Could you check a few things on this model? Use its own coordinates, in mm. A direction names the side the tool comes from. Round coordinates to 2 decimals unless told otherwise and drop trailing zeros. Order: outer loops, then holes, each group sorted by start corner. A loop starts at its lowest first (then second) coordinate and runs counter-clockwise, first axis right, second up. Notation, with made-up numbers: (-1.75, -5.75) -> (26.25, -5.75) arc R31 cw to (26.25, 32.25) -> close; hole circle Ø6 at (-18, 81.5). An arc over 180 degrees is marked (long way). One line per question, with ' | ' between items.
```python
from build123d import *

# Parameters (mm, degrees)
F0_W     = 10
F0_H     = 50
F1_DEPTH = 5.4
F3_START = 4.6
F2_W     = 8.5828267038
F2_H     = 11.0100731254
F2_W_2   = 12.8774824552
F2_H_2   = 6.9046204444
F2_W_3   = 25.3804451786
F2_H_3   = 7.8376773745
F2_H_4   = 6.3447866123
F2_W_4   = 17.729378771
F3_DEPTH = 4.8


with BuildPart() as f1:
    # F0 (on Front) → F1 (new body)
    with BuildSketch(Plane.XZ):
        Rectangle(F0_W, F0_H)
    extrude(amount=F1_DEPTH)

    # F2 (on Front) → F3 (join)
    with BuildSketch(Plane.XZ.offset(F3_START)):
        with Locations((-0.4671770148, 19.0343614668)):
            Rectangle(F2_W, F2_H)
        with Locations((10.2629775647, 19.0343614668)):
            Rectangle(F2_W_2, F2_H)
        with Locations((-0.4671770148, -7.2778436588)):
            Rectangle(F2_W, F2_H_2)
        with Locations((16.5144589264, -7.2778436588)):
            Rectangle(F2_W_3, F2_H_2)
        with Locations((-0.4671770148, -18.7544440851)):
            Rectangle(F2_W, F2_H_3)
        Polygon((3.8242363371, -14.7295454517), (3.8242363371, -14.8356053978), (3.8242363371, -22.6732827723), (43.2005375624, -22.6732827723), (43.2005375624, -14.7295454517), align=None)
        with Locations((-0.4671770148, 6.6247038776)):
            Rectangle(F2_W, F2_H_4)
        with Locations((12.6889257226, 6.6247038776)):
            Rectangle(F2_W_4, F2_H_4)
    extrude(amount=F3_DEPTH)


solid = f1.part
```
1. I want a section at C-C on y = -6.5. List the corners of the cut face in (x, z) for me.
From the geometry:
outline: (-4.76, -22.67) -> (43.2, -22.67) -> (43.2, -14.73) -> (3.82, -14.73) -> (3.82, -14.84) -> (-4.76, -14.84) -> close; (-4.76, -10.73) -> (29.2, -10.73) -> (29.2, -3.83) -> (-4.76, -3.83) -> close; (-4.76, 3.45) -> (21.55, 3.45) -> (21.55, 9.8) -> (-4.76, 9.8) -> close; (-4.76, 13.53) -> (16.7, 13.53) -> (16.7, 24.54) -> (-4.76, 24.54) -> close
2. I want a section at A-A on x = 18.5. List the corners of the cut face in (y, z) for me, and give its area (3 significant figures).
From the geometry:
outline: (-9.4, -22.67) -> (-4.6, -22.67) -> (-4.6, -14.73) -> (-9.4, -14.73) -> close; (-9.4, -10.73) -> (-4.6, -10.73) -> (-4.6, -3.83) -> (-9.4, -3.83) -> close; (-9.4, 3.45) -> (-4.6, 3.45) -> (-4.6, 9.8) -> (-9.4, 9.8) -> close | area: 102 mm²
3. I want a section at B-B on x = 13.5. List the corners of the cut face in (y, z) for me, and give its area (3 significant figures).
From the geometry:
outline: (-9.4, -22.67) -> (-4.6, -22.67) -> (-4.6, -14.73) -> (-9.4, -14.73) -> close; (-9.4, -10.73) -> (-4.6, -10.73) -> (-4.6, -3.83) -> (-9.4, -3.83) -> close; (-9.4, 3.45) -> (-4.6, 3.45) -> (-4.6, 9.8) -> (-9.4, 9.8) -> close; (-9.4, 13.53) -> (-4.6, 13.53) -> (-4.6, 24.54) -> (-9.4, 24.54) -> close | area: 155 mm²
4. I want a section at D-D on z = 21. List the corners of the cut face in (x, y) for me, and give its area (3 significant figures).
From the geometry:
outline: (-5, -5.4) -> (-4.76, -5.4) -> (-4.76, -9.4) -> (16.7, -9.4) -> (16.7, -4.6) -> (5, -4.6) -> (5, 0) -> (-5, 0) -> close | area: 149 mm²
5. If we mould it in two halves opening along Z, with no side actions, what happens to faces 1 (the face through (0, -3, 25)), 2 (the face through (16.702, -7, 19)), 3 (the face through (9, -7, 9.797)), 4 (the face through (-1, -7, -14.836))? For each: pulls with the +Z half, pulls with the -Z half, needs draft (parallel to the pull), parting line crosses it, or undercut.
From the geometry:
face 1: pulls with the +Z half | face 2: needs draft | face 3: undercut | face 4: undercut
6. I'm going to push flat-ended pins straight in: pin 1 (1.4 mm diameter, centred on x = 3, y = -6, fed in from -Z); pin 2 (2.5 mm diameter, centred on x = 23, y = -6.5, fed in from -Z); pin 3 (2 mm diameter, centred on y = -8, z = 6.5, fed in from -X); pin 4 (3.5 mm diameter, centred on x = 23, z = -8, fed in from +Y). Where does each tip first touch, or does it pass through?
From the geometry:
pin 1: stops at z = -25 | pin 2: stops at z = -22.67 | pin 3: stops at x = -4.76 | pin 4: stops at y = -4.6
7. I need wall thicknesses on probe 1 along Z at (x, y) = (19, -5.75); probe 2 along Z at (x, y) = (26.5, -7.5); probe 3 along Z at (x, y) = (16.5, -6). Which ranges of each line are inside material? Lowest first, please.
From the geometry:
probe 1: z = -22.67 to -14.73, -10.73 to -3.83, 3.45 to 9.8 | probe 2: z = -22.67 to -14.73, -10.73 to -3.83 | probe 3: z = -22.67 to -14.73, -10.73 to -3.83, 3.45 to 9.8, 13.53 to 24.54
8. On a 3-axis mill with a long thin cutter (end or side, diameter ignored), from which of +Z, -Z, +X, -X, +Y, -Y can I reach the whole of each face in a straight line? I mean faces 5 (the face through (24, -4.6, -19)), 6 (the face through (-4.759, -7, -7)), 7 (the face through (8, -7, 3.452)). Say none if no direction works.
From the geometry:
face 5: +Z, -Z, +X, +Y | face 6: +Z, -Z, -X, -Y | face 7: +X, -Y
